from build123d import *

# Parameters (mm, degrees)
SKETCH1_W           = 158
SKETCH1_H           = 158
SKETCH1_R           = 3.015623361
SKETCH1_W_2         = 109.668996446
SKETCH1_H_2         = 28.739233449
SKETCH1_W_3         = 72.233228696
SKETCH1_H_3         = 44.324935791
BOSS_EXTRUDE1_DEPTH = 3.175


with BuildPart() as part:
    # Sketch1 → Boss-Extrude1 (new body)
    with BuildSketch(Plane(origin=(0, 0, 0), x_dir=(0, 0, -1), z_dir=(1, 0, 0))):
        Rectangle(SKETCH1_W, SKETCH1_H)
        with Locations((-52.478878223, 16.641690282)):
            Circle(SKETCH1_R, mode=Mode.SUBTRACT)
        with Locations((57.521121777, 16.641690282)):
            Circle(SKETCH1_R, mode=Mode.SUBTRACT)
        with Locations((57.521121777, -50.858309718)):
            Circle(SKETCH1_R, mode=Mode.SUBTRACT)
        with Locations((-52.478878223, -50.858309718)):
            Circle(SKETCH1_R, mode=Mode.SUBTRACT)
        with Locations((0, 42.549463737)):
            Rectangle(SKETCH1_W_2, SKETCH1_H_2, mode=Mode.SUBTRACT)
        with Locations((2.521121777, -17.108309717)):
            Rectangle(SKETCH1_W_3, SKETCH1_H_3, mode=Mode.SUBTRACT)
    extrude(amount=BOSS_EXTRUDE1_DEPTH)


solid = part.part
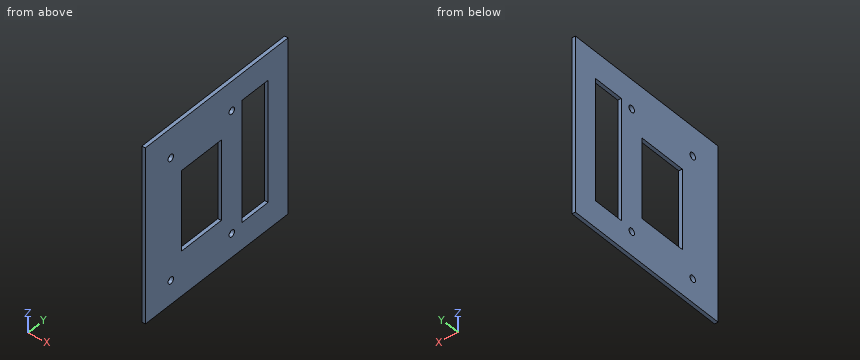
Can you work these out from the model? Positions are in its coordinate system, mm. Round coordinates to 2 decimals unless told otherwise and drop trailing zeros. Write each loop counter-clockwise with the first axis right and the second up, starting at its lowest first coordinate (ties: lowest second). Pieces come first, ordered by that corner, then holes. Notation, with made-up numbers: (61, -32.75) -> (98, -32.75) arc R13 cw to (98, -24.75) -> close; hole circle Ø1 at (-32, 43.25). An arc over 180 degrees is marked (long way). Use one line per item in the form item = value. Start each with the question number.
Q1. Imagine slicing it at D-D (x = 1.8). Please give me the cut outline in (y, z), then the cut area to 3 significant figures.
Q2. I'm going to push flat-ended pins straight in: P1, Ø12, axis at y = 2.5, z = -29, coming from the +X side (3 decimals); P2, Ø3.5, axis at y = -50.86, z = 52.48, coming from the -X side. Where does each tip first touch, or does it pass through?
Q3. Imagine slicing it at A-A (z = 5). Please give me the cut outline in (x, y) (3 decimals), then the cut area to 3 significant figures.
Q4. Imagine slicing it at B-B (y = 45). Please give me the cut outline in (x, z) (1 decimal).
Q5. If I drill on probe 1 along Y at (x, z) = (0.15, -33); probe 2 along Z at (x, y) = (0.6, 2.5); probe 3 along Y at (x, z) = (1.55, -45), over which ranges is the centre line in solid material (lowest first)? Write a range as [from, to].
Q6. Imagine slicing it at C-C (z = 42.5). Please give me the cut outline in (x, y) (3 decimals), then the cut area to 3 significant figures.
Worked out:
q1.outline = (-79, -79) -> (79, -79) -> (79, 79) -> (-79, 79) -> close; hole circle Ø6.03 at (-50.86, -57.52); hole circle Ø6.03 at (-50.86, 52.48); hole (-39.27, -38.64) -> (5.05, -38.64) -> (5.05, 33.6) -> (-39.27, 33.6) -> close; hole circle Ø6.03 at (16.64, -57.52); hole circle Ø6.03 at (16.64, 52.48); hole (28.18, -54.83) -> (56.92, -54.83) -> (56.92, 54.83) -> (28.18, 54.83) -> close
q1.area = 18,500 mm^2
q2.P1 = 3.175
q2.P2 = through
q3.outline = (0, -79) -> (3.175, -79) -> (3.175, -39.271) -> (0, -39.271) -> close; (0, 5.054) -> (3.175, 5.054) -> (3.175, 28.18) -> (0, 28.18) -> close; (0, 56.919) -> (3.175, 56.919) -> (3.175, 79) -> (0, 79) -> close
q3.area = 270 mm^2
q4.outline = (0, -79) -> (3.2, -79) -> (3.2, -54.8) -> (0, -54.8) -> close; (0, 54.8) -> (3.2, 54.8) -> (3.2, 79) -> (0, 79) -> close
q5.probe_1 = [-79, -39.27], [5.05, 28.18], [56.92, 79]
q5.probe_2 = [-79, -38.64], [33.6, 79]
q5.probe_3 = [-79, 28.18], [56.92, 79]
q6.outline = (0, -79) -> (3.175, -79) -> (3.175, 28.18) -> (0, 28.18) -> close; (0, 56.919) -> (3.175, 56.919) -> (3.175, 79) -> (0, 79) -> close
q6.area = 410 mm^2
